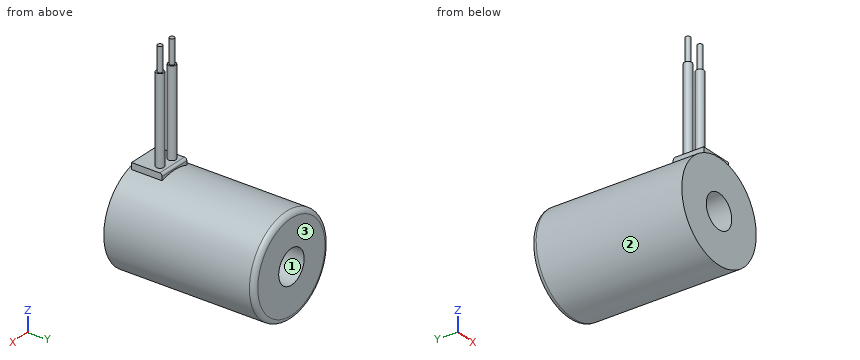
from build123d import *

# Parameters (mm, degrees)
BASE_SKETCH_R       = 10.25
BASE_EXTRUDE_DEPTH  = 15.7
BODY_FILLET_R       = 1
WIRE_BASE_SKETCH_W  = 6.8
WIRE_BASE_SKETCH_H  = 6.4
WIRE_BASE_DEPTH     = 11
WIRE_BASE_FILLET_R  = 0.5
WIRE_START_SKETCH_R = 0.8
WIRE_START_DEPTH    = 18
WIRE_END_SKETCH_R   = 0.5
WIRE_END_DEPTH      = 5
THRU_HOLE_SKETCH_R  = 3.5
THRU_HOLE_DEPTH     = 48.402768906


with BuildPart() as part:
    # Base Sketch → Base Extrude (new, symmetric)
    with BuildSketch(Plane(origin=(0, 0, 0), x_dir=(1, 0, 0), z_dir=(0, 1, 0))):
        with Locations(Location((0, 0, 0), (0, 0, 270))):
            Circle(BASE_SKETCH_R)
    extrude(amount=BASE_EXTRUDE_DEPTH, both=True)

    # Body Fillet
    body_fillet_edges = [part.edges().sort_by_distance(p)[0] for p in [
        (0, 15.7, -10.25),
    ]]
    fillet(body_fillet_edges, radius=BODY_FILLET_R)

    # Wire Base Sketch → Wire Base (add)
    with BuildSketch(Plane.XY):
        with Locations((0, -11.9)):
            Rectangle(WIRE_BASE_SKETCH_W, WIRE_BASE_SKETCH_H)
    extrude(amount=WIRE_BASE_DEPTH)

    # Wire Base Fillet
    wire_base_fillet_edges = [part.edges().sort_by_distance(p)[0] for p in [
        (0, -8.7, 11),
    ]]
    fillet(wire_base_fillet_edges, radius=WIRE_BASE_FILLET_R)

    # Wire Start Sketch → Wire Start (add)
    with BuildSketch(Plane.XY.offset(11)):
        with Locations((-1.8, -10.6)):
            Circle(WIRE_START_SKETCH_R)
        with Locations((1.5, -10.6)):
            Circle(WIRE_START_SKETCH_R)
    extrude(amount=WIRE_START_DEPTH)

    # Wire End Sketch → Wire End (add)
    with BuildSketch(Plane.XY.offset(29)):
        with Locations((1.5, -10.6)):
            Circle(WIRE_END_SKETCH_R)
        with Locations((-1.8, -10.6)):
            Circle(WIRE_END_SKETCH_R)
    extrude(amount=WIRE_END_DEPTH)

    # Thru Hole Sketch → Thru Hole (cut, through all)
    with BuildSketch(Plane(origin=(0, 15.7, 0), x_dir=(1, 0, 0), z_dir=(0, 1, 0))):
        with Locations(Location((0, 0, 0), (0, 0, 270))):
            Circle(THRU_HOLE_SKETCH_R)
    extrude(amount=-THRU_HOLE_DEPTH, mode=Mode.SUBTRACT)


solid = part.part
Source: CAD feature listing. Evaluate the final solid. Frame: model axes, mm. Face numbers are marked on the shaded views. Coordinates: 2 decimals unless noted, no trailing zeros. Order: outer loops, then holes, each group sorted by start corner. A loop starts at its lowest first (then second) coordinate and runs counter-clockwise, first axis right, second up.
Item 1: Cut plane B-B (z = 0). Return loops of the section in (x, y).
Output values:
outline: (-10.25, -15.7) - (-3.5, -15.7) - (-3.5, 15.7) - (-9.25, 15.7) arc R1 ccw to (-10.25, 14.7) - close; (3.5, -15.7) - (10.25, -15.7) - (10.25, 14.7) arc R1 ccw to (9.25, 15.7) - (3.5, 15.7) - close
Item 2: First-contact query: P1, Ø2, axis at y = -1, z = -1.5, coming from the -X side; P2, Ø4, axis at x = -5.5, y = -10.5, coming from the -Z side; P3, Ø8, axis at x = -3, y = 9.5, coming from the +Z side. Flat tips, straight axial feed; report the tip coordinate or a pass-through.
Output values:
P1: stops at x = -10.24
P2: stops at z = -9.63
P3: stops at z = 10.25
Item 3: Material intervals for line 1 (X direction, y = -4.5, z = 0); line 2 (Z direction, x = -1.5, y = 6.5); line 3 (Z direction, x = -2, y = -3), sorted ascending.
Output values:
line 1: x = -10.25 to -3.5, 3.5 to 10.25
line 2: z = -10.14 to -3.16, 3.16 to 10.14
line 3: z = -10.05 to -2.87, 2.87 to 10.05
Item 4: Cut plane C-C (y = -10.6). Return loops of the section in (x, z).
Output values:
outline: (-3.4, 9.67) arc R10.25 ccw (long way) to (3.4, 9.67) - (3.4, 11) - (2.3, 11) - (2.3, 29) - (2, 29) - (2, 34) - (1, 34) - (1, 29) - (0.7, 29) - (0.7, 11) - (-1, 11) - (-1, 29) - (-1.3, 29) - (-1.3, 34) - (-2.3, 34) - (-2.3, 29) - (-2.6, 29) - (-2.6, 11) - (-3.4, 11) - close; hole circle Ø7 at (0, 0)
Item 5: Cut plane A-A (x = 0). Return loops of the section in (y, z).
Output values:
outline: (-15.7, -10.25) - (14.7, -10.25) arc R1 ccw to (15.7, -9.25) - (15.7, -3.5) - (-15.7, -3.5) - close; (-15.7, 3.5) - (15.7, 3.5) - (15.7, 9.25) arc R1 ccw to (14.7, 10.25) - (-8.7, 10.25) - (-8.7, 10.5) arc R0.5 ccw to (-9.2, 11) - (-15.1, 11) - (-15.1, 10.25) - (-15.7, 10.25) - close
Item 6: Cut plane D-D (z = 31). Return loops of the section in (x, y), plus the area to 3 significant figures.
Output values:
outline: circle Ø1 at (-1.8, -10.6); circle Ø1 at (1.5, -10.6)
area: 1.57 mm2
Item 7: Pull-direction query (Z, two-part tool) for the marked faces 1, 2 and 3; classes: pulls with the +Z half, pulls with the -Z half, needs draft (parallel to the pull), parting line crosses it, or undercut.
Output values:
face 1: undercut
face 2: parting line crosses it
face 3: needs draft
